Verification items for the finished model (mm, model axes). Face numbers are marked on the shaded views. A direction names the side the tool comes from. Coordinates: 2 decimals unless noted, no trailing zeros. Loops run counter-clockwise (first coordinate to the right, second up) from the corner with the lowest first, then second, coordinate; pieces in that order, holes last. Notation, with made-up numbers: (-0.75, 30.5) -> (35.25, 30.5) arc R15 cw to (35.25, 56.5) -> close; hole circle Ø5 at (40.25, 3.25). An arc over 180 degrees is marked (long way). Answer as a JSON object with one key per item and string values. Group by question number.
Q1. Set-up check for the marked faces 1, 2 and 3: record each of +Z, -Z, +X, -X, +Y, -Y from which the full face is reachable in a straight line by a thin tool's end or side.
Q2. Scan lines: L1, parallel to Z at x = 1.5, y = 4.25; L2, parallel to X at y = 4.25, z = -4.5; L3, parallel to Y at x = 11.5, z = -1. Record each from-to range of solid material in increasing order.
Q3. Cross-section at D-D on z = -3. Record the boundary of the cut face in (x, y), and give its area (3 significant figures).
Q4. Cross-section at C-C on y = 2.75. Record the boundary of the cut face in (x, z), and give its area (3 significant figures).
Q5. Cross-section at A-A on x = 7.75. Record the boundary of the cut face in (y, z).
Q6. Gauge pin test, flat ends, axial feed: pin 1 Ø2 at (x, y) = (9, 7) entering from +Z; pin 2 Ø1 at (x, z) = (12, -12.5) entering from +Y; pin 3 Ø0.9 at (x, y) = (7.5, 3.5) entering from -Z. Record the tip position at first contact, or that the pin passes through.
Q7. Cross-section at B-B on z = -5. Record the boundary of the cut face in (x, y).
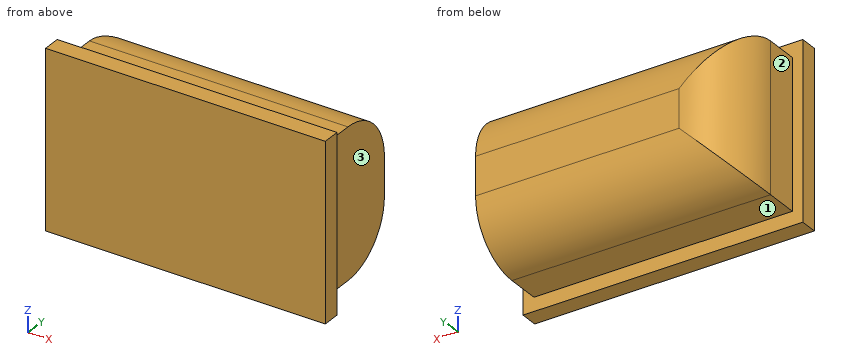
```python
from build123d import *

# Parameters (mm, degrees)
SKETCH1_W           = 25.4
SKETCH1_H           = 16
BOSS_EXTRUDE1_DEPTH = 1.6
SKETCH2_W           = 23.471528358
SKETCH2_H           = 13.466700145
BOSS_EXTRUDE2_DEPTH = 8
FILLET1_R           = 5


with BuildPart() as part:
    # Sketch1 → Boss-Extrude1 (new body)
    with BuildSketch(Plane(origin=(0, 0, 0), x_dir=(1, 0, 0), z_dir=(0, 1, 0))):
        with Locations((12.7, 8)):
            Rectangle(SKETCH1_W, SKETCH1_H)
    extrude(amount=BOSS_EXTRUDE1_DEPTH)

    # Sketch2 → Boss-Extrude2 (add)
    with BuildSketch(Plane(origin=(0, 1.6, 0), x_dir=(1, 0, 0), z_dir=(0, 1, 0))):
        with Locations((12.677642984, 8.013617828)):
            Rectangle(SKETCH2_W, SKETCH2_H)
    extrude(amount=BOSS_EXTRUDE2_DEPTH)

    # Fillet1
    fillet1_edges = [part.edges().sort_by_distance(p)[0] for p in [
        (0.941878805, 9.6, -8.013617827),
        (12.677642984, 9.6, -1.280267755),
        (12.677642984, 9.6, -14.7469679),
    ]]
    fillet(fillet1_edges, radius=FILLET1_R)


solid = part.part
```
Computed values:
{
 "1": {"face 1": "-Z, +X, -X, +Y", "face 2": "+Z, -Z, -X, +Y", "face 3": "+Z, -Z, +X, +Y"},
 "2": {"L1": "z = -14.75 to -1.28", "L2": "x = 0.94 to 24.41", "L3": "y = 0 to 1.6"},
 "3": {"outline": "(0, 0) -> (25.4, 0) -> (25.4, 1.6) -> (24.41, 1.6) -> (24.41, 8.37) -> (2.66, 8.37) arc R5 ccw to (0.94, 4.6) -> (0.94, 1.6) -> (0, 1.6) -> close", "area": "198 mm²"},
 "4": {"outline": "(0.94, -14.75) -> (24.41, -14.75) -> (24.41, -1.28) -> (0.94, -1.28) -> close", "area": "316 mm²"},
 "5": {"outline": "(0, -16) -> (1.6, -16) -> (1.6, -14.75) -> (4.6, -14.75) arc R5 ccw to (9.6, -9.75) -> (9.6, -6.28) arc R5 ccw to (4.6, -1.28) -> (1.6, -1.28) -> (1.6, 0) -> (0, 0) -> close"},
 "6": {"pin 1": "stops at z = -1.48", "pin 2": "stops at y = 9.06", "pin 3": "stops at z = -14.75"},
 "7": {"outline": "(0, 0) -> (25.4, 0) -> (25.4, 1.6) -> (24.41, 1.6) -> (24.41, 9.43) -> (4.66, 9.43) arc R5 ccw to (0.94, 4.6) -> (0.94, 1.6) -> (0, 1.6) -> close"}
}
